Part model, mm, in its own coordinate system. A direction names the side the tool comes from. Coordinates: 2 decimals unless noted, no trailing zeros. Loops run counter-clockwise (first coordinate to the right, second up) from the corner with the lowest first, then second, coordinate; pieces in that order, holes last. Notation, with made-up numbers: M 46.5,4.5 L 81.5,4.5 A14 cw 81.5,16.5 Z; hole C 50,15 d2. An arc over 180 degrees is marked long. Answer as a JSON object with one key per item and string values. Group by question number.
1. Saw through at D-D on y = 92. Write the cut outline in (x, z).
2. 3-axis set-ups, long thin cutter, end or side, ignore diameter. For faces 5 (the face through (-21, -12.967, -24)), 6 (the face through (-27.8, -6.2, -24.1)), 7 (the face through (-26, -15, -24)): which of +Z, -Z, +X, -X, +Y, -Y reach the whole face in a straight line?
3. Mould opens along Y. For faces 1 (the face through (-28.32, 0, -24)), 2 (the face through (-45, -18.967, -24)), 3 (the face through (-83.492, 83, -21)), 4 (the face through (-88.12, 123.924, -17.777)) say: released by +Y, released by -Y, zero draft, split by the parting line, or undercut.
4. Drop flat-ended pins along their axis: pin 1 Ø5.5 at (x, z) = (-21, -24) entering from +Y; pin 2 Ø6.5 at (y, z) = (-1.5, -22.5) entering from +X; pin 3 Ø10 at (y, z) = (86.5, -28.5) entering from -X; pin 4 Ø5 at (y, z) = (34, -31.5) entering from +X. Give the stop position or say it passes through.
5. Saw through at B-B on x = -50. Write the cut outline in (y, z).
6. Drill centre lines: L1, parallel to X at y = 45.5, z = -28.75; L2, parallel to Y at x = -33, z = -29.5; L3, parallel to Y at x = -86.75, z = -19 (3 decimals). Where is each one in solid material? Low to high.
Autodesk Inventor part; units mm, degrees
ref_plane "YZ Plane" through (0, 0, 0) normal (1, 0, 0) x (0, 1, 0)
ref_plane "XZ Plane" through (0, 0, 0) normal (0, 1, 0) x (-1, 0, 0)
ref_plane "XY Plane" through (0, 0, 0) normal (0, 0, 1) x (1, 0, 0)
ref_plane "Work Plane1" through (0, 0, 0) normal (0, 0, 1) x (1, 0, 0)
ref_plane "Work Plane2" through (0, 0, -24) normal (0, 0, 1) x (1, 0, 0)
sketch "Sketch1" plane through (0, 0, -24) normal (0, 0, 1) x (1, 0, 0)
  line L0 (-28.32, -15) -> (-28.32, -9.975)
  line L1 (-28.32, -3.975) -> (-28.32, 4.075)
  line L2 (-23.82, -15) -> (-28.32, -15)
  line L3 (-23.82, -15) -> (-23.52, -15)
  line L4 (-23.52, -15) -> (-23.82, -12.9669)
  line L5 (-23.82, -12.9669) -> (-18.8601, -12.9669)
  line L6 (-18.8601, -12.9669) -> (-18.8601, -18.9669)
  line L7 (-18.8601, -18.9669) -> (-92.6205, -18.9669)
  line L8 (-92.6205, -18.9669) -> (-92.6205, 137.182)
  line L9 (-92.6205, 137.182) -> (-83.4923, 137.182)
  line L10 (-83.4923, 137.182) -> (-83.4923, 6.5025)
  line L11 (-83.4923, 6.5025) -> (-28.32, 6.5025)
  line L12 (-28.32, -3.975) -> (-26.9128, -9.975)
  line L13 (-26.9128, -9.975) -> (-28.4348, -9.773)
  line L14 (-28.4348, -9.773) -> (-28.32, -10.5507)
  line L15 (-28.32, -10.5507) -> (-28.32, -15)
  line L16 (-28.32, -15) -> (-23.82, -15)
  line L17 (-28.32, 4.075) -> (-28.32, 4.2239)
  line L18 (-28.32, 4.2239) -> (-26.4709, 4.2239)
  line L19 (-26.4709, 4.2239) -> (-26.4709, 6.5025)
  line L20 (-26.4709, 6.5025) -> (-28.32, 6.5025)
  point P0 (0, 0)
  dimension "d0" = 0.3
  dimension "d1" = 6
extrude "Extrusion1" add sketch "Sketch1" along normal mid plane 20
fillet "Fillet1" radius 1 1 edges at (-26.9128, -9.975, -24)
chamfer "Chamfer1" distance 20 angle 45 2 edges at (-83.4923, 6.5025, -24) (-92.6205, -18.9669, -24)
sketch "Sketch2" plane through (-92.6205, 137.182, -34) normal (-1, 0, 0) x (0, 0, 1)
  line L0 (18.675, -27.877) -> (18.675, 6.063)
  line L1 (-16.4278, 9.4711) -> (-17.2496, 12.5384)
  line L2 (-17.2496, 12.5384) -> (-20.3169, 13.3602)
  line L3 (-20.3169, 13.3602) -> (-22.5622, 11.1149)
  line L4 (-22.5622, 11.1149) -> (-21.7404, 8.0476)
  line L5 (-21.7404, 8.0476) -> (-18.6731, 7.2258)
  line L6 (-18.6731, 7.2258) -> (-16.4278, 9.4711)
  line L7 (23.7269, -35.1742) -> (25.9722, -32.9289)
  line L8 (25.9722, -32.9289) -> (25.1504, -29.8616)
  line L9 (25.1504, -29.8616) -> (22.0831, -29.0398)
  line L10 (22.0831, -29.0398) -> (19.8378, -31.2851)
  line L11 (19.8378, -31.2851) -> (20.6596, -34.3524)
  line L12 (20.6596, -34.3524) -> (23.7269, -35.1742)
  circle A0 centre (16.005, 9.753) radius 2.475
  circle A1 centre (-18.955, 3.393) radius 2.475
  circle A2 centre (-12.595, -31.567) radius 2.475
  circle A3 centre (22.365, -25.207) radius 2.475
  circle A4 centre (22.365, 3.393) radius 2.475
  circle A5 centre (16.005, -31.567) radius 2.475
  circle A6 centre (-18.955, -25.207) radius 2.475
  circle A7 centre (-12.595, 9.753) radius 2.475
  arc A8 (-20.655, -19.707) -> (-17.255, -19.707) centre (-18.955, -19.707) ccw
  line L13 (-17.255, -19.707) -> (-17.255, -2.107)
  arc A9 (-17.255, -2.107) -> (-20.655, -2.107) centre (-18.955, -2.107) ccw
  line L14 (-20.655, -2.107) -> (-20.655, -19.707)
  arc A10 (20.665, -19.707) -> (24.065, -19.707) centre (22.365, -19.707) ccw
  line L15 (24.065, -19.707) -> (24.065, -2.107)
  arc A11 (24.065, -2.107) -> (20.665, -2.107) centre (22.365, -2.107) ccw
  line L16 (20.665, -2.107) -> (20.665, -19.707)
  arc A12 (10.505, -33.267) -> (10.505, -29.867) centre (10.505, -31.567) ccw
  line L17 (10.505, -29.867) -> (-7.095, -29.867)
  arc A13 (-7.095, -29.867) -> (-7.095, -33.267) centre (-7.095, -31.567) ccw
  line L18 (-7.095, -33.267) -> (10.505, -33.267)
  arc A14 (-7.095, 11.453) -> (-7.095, 8.053) centre (-7.095, 9.753) ccw
  line L19 (-7.095, 8.053) -> (10.505, 8.053)
  arc A15 (10.505, 8.053) -> (10.505, 11.453) centre (10.505, 9.753) ccw
  line L20 (10.505, 11.453) -> (-7.095, 11.453)
  line L21 (-15.265, -27.877) -> (18.675, -27.877)
  line L22 (18.675, -27.877) -> (18.675, 6.063)
  line L23 (18.675, 6.063) -> (-15.265, 6.063)
  line L24 (-15.265, 6.063) -> (-15.265, -27.877)
  circle A16 centre (-19.495, -32.107) radius 2.75
  circle A17 centre (22.905, 10.293) radius 2.75
  arc A18 (-22.645, -33.757) -> (-21.145, -35.257) centre (-21.145, -33.757) ccw
  line L25 (-22.645, 11.943) -> (-22.645, -33.757)
  arc A19 (-21.145, 13.443) -> (-22.645, 11.943) centre (-21.145, 11.943) ccw
  line L26 (24.555, 13.443) -> (-21.145, 13.443)
  arc A20 (26.055, 11.943) -> (24.555, 13.443) centre (24.555, 11.943) ccw
  line L27 (26.055, -33.757) -> (26.055, 11.943)
  arc A21 (24.555, -35.257) -> (26.055, -33.757) centre (24.555, -33.757) ccw
  line L28 (-21.145, -35.257) -> (24.555, -35.257)
  circle A22 centre (1.705, -10.907) radius 16.97
  circle A23 centre (15, -10.907) radius 2.65
  line L29 (20, 0) -> (20, -136.1489)
  line L30 (20, -136.1489) -> (0, -136.1489)
  line L31 (20, 0) -> (20, -136.1489)
  line L32 (0, 0) -> (20, 0)
  line L33 (0, -136.1489) -> (0, 0)
  line L34 (0, 0) -> (20, 0)
  line L35 (10, 0) -> (0, -136.1489)
  point P0 (34, -137.182)
  dimension "d8" = 5.3
  dimension "d9" = 5
extrude "Extrusion2" cut sketch "Sketch2" against normal through all contours L35 L17 L33 L21 | L21 A22 L35 | A22 L33 L32 L35 | L21 L33 A22 | L35 L18 L33 L17 | L35 L28 L33 L18 | L35 L33 L28 | A23
properties part number "30_Adapter_neje_LED"
Outcome:
{
 "1": {"outline": "M -92.62,-27.32 L -83.49,-27.32 L -83.49,-14 L -92.62,-14 Z"},
 "2": {"face 5": "+Z, -Z, +X, +Y", "face 6": "+Z, -Z, +X", "face 7": "+Z, -Z"},
 "3": {"face 1": "undercut", "face 2": "released by -Y", "face 3": "zero draft", "face 4": "undercut"},
 "4": {"pin 1": "stops at y = -12.97", "pin 2": "stops at x = -28.14", "pin 3": "stops at x = -92.62", "pin 4": "stops at x = -83.49"},
 "5": {"outline": "M -18.97,-34 L 1.03,-34 L 6.5,-33.6 L 6.5,-14 L -18.97,-14 Z"},
 "6": {"L1": "x = -92.62 to -83.49", "L2": "y = -18.97 to 6.5", "L3": "y = -4.837 to 123.625, 128.925 to 137.182"}
}
